```python
from build123d import *

# Parameters (mm, degrees)
CHAMFER_1_SIZE = 1


with BuildPart() as part:
    # Sketch 1 → Revolve 1 (revolve)
    with BuildSketch(Plane.XY, mode=Mode.PRIVATE) as revolve_1_sk:
        with BuildLine():
            Line((-22.2, 27.5), (33.4, 27.5))
            Line((33.4, 27.5), (33.4, 36.1))
            Line((33.4, 36.1), (3.6, 36.1))
            ThreePointArc((3.6, 36.1), (0, 34.3), (-3.6, 36.1))
            Line((-3.6, 36.1), (-22.2, 36.1))
            Line((-22.2, 36.1), (-22.2, 27.5))
        make_face()
    revolve(revolve_1_sk.sketch.rotate(Axis((-55.01659168, 0, 0), (1, 0, 0)), 90), axis=Axis((-55.01659168, 0, 0), (1, 0, 0)))

    # Chamfer 1
    chamfer_1_edges = [part.edges().sort_by_distance(p)[0] for p in [
        (-22.2, 0, -36.1),
        (33.4, 0, -36.1),
        (33.4, 0, -27.5),
        (-22.2, 0, -27.5),
    ]]
    chamfer(chamfer_1_edges, length=CHAMFER_1_SIZE)


solid = part.part
```
Can you work these out from the model? Positions are in its coordinate system, mm. Give positions to 0.01 mm unless a question says otherwise; leave off trailing zeros. Order: outer loops, then holes, each group sorted by start corner. A loop starts at its lowest first (then second) coordinate and runs counter-clockwise, first axis right, second up. Notation, with made-up numbers: M 45,-32.5 L 56,-32.5 A21 ccw 56,-10.5 Z; hole C 20,54.5 d2. An arc over 180 degrees is marked long. Write item = value, one per line. Start each with the question number.
Q1. I need wall thicknesses on probe 1 along Y at (x, z) = (-5, 0); probe 2 along Z at (x, y) = (-19, 1); probe 3 along Y at (x, z) = (26, -5). Which ranges of each line are inside material? Lowest first, please. Write a range as [from, to].
Q2. Will these pins go through, and if not, where does the flat tip stop? pin 1 Ø3 at (x, y) = (-4, 12) entering from -Z; pin 2 Ø1.5 at (x, y) = (-4, 13.5) entering from +Z; pin 3 Ø2 at (y, z) = (8.5, 25) entering from -X; pin 4 Ø1 at (x, y) = (-14.5, -16) entering from +Z.
Q3. Suppose I cut it at A-A (z = 0). Write out the boundary of the cut face in (x, y).
Q4. Suppose I cut it at C-C (x = -16). Write out the boundary of the cut face in (y, z).
Q5. We'd pull the mould along Z, two halves only. Please class faces 1 (the flat face through (-22.2, -29, 0)), 2 (the cylindrical face through (17.798, 21.966, -28.648)), 3 (the cylindrical face through (5.975, 24.397, 12.69)): pulls with the +Z half, pulls with the -Z half, needs draft (parallel to the pull), parting line crosses it, or undercut.
Check result:
q1.probe_1 = [-36.1, -27.5], [27.5, 36.1]
q1.probe_2 = [-36.09, -27.48], [27.48, 36.09]
q1.probe_3 = [-35.75, -27.04], [27.04, 35.75]
q2.pin_1 = -34.54
q2.pin_2 = 33.77
q2.pin_3 = through
q2.pin_4 = 32.6
q3.outline = M -22.2,-35.1 L -21.2,-36.1 L -3.6,-36.1 A4.5 cw 3.6,-36.1 L 32.4,-36.1 L 33.4,-35.1 L 33.4,-28.5 L 32.4,-27.5 L -21.2,-27.5 L -22.2,-28.5 Z; M -22.2,28.5 L -21.2,27.5 L 32.4,27.5 L 33.4,28.5 L 33.4,35.1 L 32.4,36.1 L 3.6,36.1 A4.5 cw -3.6,36.1 L -21.2,36.1 L -22.2,35.1 Z
q4.outline = C 0,0 d72.2; hole C 0,0 d55
q5.face_1 = needs draft
q5.face_2 = parting line crosses it
q5.face_3 = undercut
